Could you check a few things on this model? Use its own coordinates, in mm. A direction names the side the tool comes from. Coordinates: 2 decimals unless noted, no trailing zeros. Loops run counter-clockwise (first coordinate to the right, second up) from the corner with the lowest first, then second, coordinate; pieces in that order, holes last.
from build123d import *

# Parameters (mm, degrees)
SKETCH1_W           = 320
SKETCH1_H           = 250
SKETCH1_R           = 10
BOSS_EXTRUDE1_DEPTH = 20
SKETCH2_R           = 7.5
CUT_EXTRUDE1_DEPTH  = 205.022057631
FILLET1_R           = 70
BOSS_EXTRUDE2_DEPTH = 175


# Read off the part's stored shape, not the designer's step: Boss-Extrude2
with BuildPart() as part:
    # Sketch1 → Boss-Extrude1 (new body)
    with BuildSketch(Plane.XY):
        Rectangle(SKETCH1_W, SKETCH1_H)
        with Locations((62.5, 0)):
            Circle(SKETCH1_R, mode=Mode.SUBTRACT)
        with Locations((-62.5, 0)):
            Circle(SKETCH1_R, mode=Mode.SUBTRACT)
    extrude(amount=BOSS_EXTRUDE1_DEPTH)

    # Sketch2 → Cut-Extrude1 (cut, through all)
    with BuildSketch(Plane.XY.offset(20)):
        with Locations((0, 90.519334951)):
            Circle(SKETCH2_R)
        with Locations((-125, 90.519334951)):
            Circle(SKETCH2_R)
        with Locations((125, 90.519334951)):
            Circle(SKETCH2_R)
    extrude(amount=-CUT_EXTRUDE1_DEPTH, mode=Mode.SUBTRACT)

    # Fillet1
    fillet1_edges = [part.edges().sort_by_distance(p)[0] for p in [
        (160, -125, 10),
        (-160, -125, 10),
    ]]
    fillet(fillet1_edges, radius=FILLET1_R)

    # Boss-Extrude2 outline → Boss-Extrude2 (add)
    with BuildSketch(Plane(origin=(0, 0, 0), x_dir=(-1, 0, 0), z_dir=(0, 0, -1))):
        with BuildLine():
            Line((-90, -125), (90, -125))
            ThreePointArc((90, -125), (139.497474683, -104.497474683), (160, -55))
            Line((160, -55), (145, -55))
            ThreePointArc((145, -55), (128.890872965, -93.890872965), (90, -110))
            Line((90, -110), (-90, -110))
            ThreePointArc((-90, -110), (-128.890872965, -93.890872965), (-145, -55))
            Line((-145, -55), (-160, -55))
            ThreePointArc((-160, -55), (-139.497474683, -104.497474683), (-90, -125))
        make_face()
    extrude(amount=BOSS_EXTRUDE2_DEPTH)


solid = part.part
(1) Which directions (+Z, -Z, +X, -X, +Y, -Y) give clear straight access to the entire face, cutting with the end or side of a thin tool? Please do faces 1 (the face through (-1, -110, -86)), 2 (the face through (160, 34, 10)), 3 (the face through (-153, -55, -86)).
Answers:
face 1: -Z, +Y
face 2: +Z, -Z, +X, +Y, -Y
face 3: -Z, +X, -X, +Y
(2) Imagine slicing it at D-D, the plane y = -79.5. Write out the boundary of the cut face in (x, z), and give its area (3 significant figures).
Answers:
outline: (-155.57, -175) - (-139.24, -175) - (-139.24, 0) - (139.24, 0) - (139.24, -175) - (155.57, -175) - (155.57, 20) - (-155.57, 20) - close
area: 11,900 mm2
(3) For pin 1 (23 mm diameter, centred on x = 62.5, y = 0, fed in from -Z); pin 2 (3 mm diameter, centred on y = -7.5, z = -1, fed in from -X); pin 3 (12 mm diameter, centred on x = 152.5, z = -54, fed in from +Y); pin 4 (2 mm diameter, centred on x = -106, z = -59.5, fed in from +Y), each with a flat end and sliding along its axis, tell me the tip position at first contact or that it passes through.
Answers:
pin 1: stops at z = 0
pin 2: stops at x = -160
pin 3: stops at y = -55
pin 4: stops at y = -107.31
(4) We'd pull the mould along Y, two halves only. Please class faces 4 (the face through (-129.316, -93.461, -86.275)), 5 (the face through (1, -111, -175)), 6 (the face through (-1.63, 83.2, 10.14)): +Y half, -Y half, draft (parallel to the pull), parting line (faces both ways), or undercut.
Answers:
face 4: +Y half
face 5: draft
face 6: undercut
(5) Imagine slicing it at C-C, the plane x = 62.5. Write out the boundary of the cut face in (y, z), and give its area (4 significant figures).
Answers:
outline: (-125, -175) - (-110, -175) - (-110, 0) - (-10, 0) - (-10, 20) - (-125, 20) - close; (10, 0) - (125, 0) - (125, 20) - (10, 20) - close
area: 7,225 mm2
(6) Imagine slicing it at B-B, the plane z = -25. Write out the boundary of the cut face in (x, y).
Answers:
outline: (-160, -55) arc R70 ccw to (-90, -125) - (90, -125) arc R70 ccw to (160, -55) - (145, -55) arc R55 cw to (90, -110) - (-90, -110) arc R55 cw to (-145, -55) - close
(7) I need wall thicknesses on probe 1 along Y at (x, z) = (-62, 5); probe 2 along Y at (x, z) = (0, 10.75); probe 3 along Z at (x, y) = (21, -13.5). Which ranges of each line are inside material? Lowest first, please.
Answers:
probe 1: y = -125 to -9.99, 9.99 to 125
probe 2: y = -125 to 83.02, 98.02 to 125
probe 3: z = 0 to 20
(8) Imagine slicing it at A-A, the plane x = 0. Write out the boundary of the cut face in (y, z).
Answers:
outline: (-125, -175) - (-110, -175) - (-110, 0) - (83.02, 0) - (83.02, 20) - (-125, 20) - close; (98.02, 0) - (125, 0) - (125, 20) - (98.02, 20) - close
